Part model, mm, in its own coordinate system. A direction names the side the tool comes from. Give positions to 0.01 mm unless a question says otherwise; leave off trailing zeros. Write each loop counter-clockwise with the first axis right and the second up, starting at its lowest first coordinate (ties: lowest second). Pieces come first, ordered by that corner, then holes.
from build123d import *

# Parameters (mm, degrees)
SKETCH_1_R          = 4.75
EXTRUDE_1_DEPTH     = 7
SKETCH_2_R          = 6.5
EXTRUDE_2_DEPTH     = 1
SKETCH_3_R          = 6.5
EXTRUDE_3_DEPTH     = 1
SKETCH_4_R          = 1.5
CUT_EXTRUDE_1_DEPTH = 12
SKETCH_5_R          = 4
SKETCH_5_R_2        = 2
CUT_EXTRUDE_2_DEPTH = 0.5
SKETCH_6_R          = 4
SKETCH_6_R_2        = 2
CUT_EXTRUDE_3_DEPTH = 0.5


with BuildPart() as part:
    # 草图1 → 凸台-拉伸1 (new body)
    with BuildSketch(Plane.XY):
        Circle(SKETCH_1_R)
    extrude(amount=EXTRUDE_1_DEPTH)

    # 草图2 → 凸台-拉伸2 (add)
    with BuildSketch(Plane.XY.offset(7)):
        Circle(SKETCH_2_R)
    extrude(amount=EXTRUDE_2_DEPTH)

    # 草图3 → 凸台-拉伸3 (add)
    with BuildSketch(Plane(origin=(0, 0, 0), x_dir=(-1, 0, 0), z_dir=(0, 0, -1))):
        Circle(SKETCH_3_R)
    extrude(amount=EXTRUDE_3_DEPTH)

    # 草图4 → 切除-拉伸1 (cut)
    with BuildSketch(Plane(origin=(0, 0, -1), x_dir=(-1, 0, 0), z_dir=(0, 0, -1))):
        Circle(SKETCH_4_R)
    extrude(amount=-CUT_EXTRUDE_1_DEPTH, mode=Mode.SUBTRACT)

    # 草图5 → 切除-拉伸2 (cut)
    with BuildSketch(Plane(origin=(0, 0, -1), x_dir=(-1, 0, 0), z_dir=(0, 0, -1))):
        Circle(SKETCH_5_R)
        Circle(SKETCH_5_R_2, mode=Mode.SUBTRACT)
    extrude(amount=-CUT_EXTRUDE_2_DEPTH, mode=Mode.SUBTRACT)

    # 草图6 → 切除-拉伸3 (cut)
    with BuildSketch(Plane.XY.offset(8)):
        Circle(SKETCH_6_R)
        Circle(SKETCH_6_R_2, mode=Mode.SUBTRACT)
    extrude(amount=-CUT_EXTRUDE_3_DEPTH, mode=Mode.SUBTRACT)


solid = part.part
1) Drill centre lines: L1, parallel to Y at x = 0, z = -0.65; L2, parallel to Z at x = 3.75, y = -5; L3, parallel to Y at x = 0, z = 1. Where is each one in solid material? Low to high.
Check result:
L1: y = -6.5 to -4, -2 to -1.5, 1.5 to 2, 4 to 6.5
L2: z = -1 to 0, 7 to 8
L3: y = -4.75 to -1.5, 1.5 to 4.75
2) Saw through at C-C (x = 2.5). Write the cut outline in (y, z).
Check result:
outline: (-6, -1) - (-3.12, -1) - (-3.12, -0.5) - (3.12, -0.5) - (3.12, -1) - (6, -1) - (6, 0) - (4.04, 0) - (4.04, 7) - (6, 7) - (6, 8) - (3.12, 8) - (3.12, 7.5) - (-3.12, 7.5) - (-3.12, 8) - (-6, 8) - (-6, 7) - (-4.04, 7) - (-4.04, 0) - (-6, 0) - close
3) 3-axis set-ups, long thin cutter, end or side, ignore diameter. For faces 1 (the flat face through (0, -5, 0)), 2 (the flat face through (2, -1, -0.5)), 3 (the cylindrical face through (-0.434, -1.952, 7.754)): which of +Z, -Z, +X, -X, +Y, -Y reach the whole face in a straight line?
Check result:
face 1: none
face 2: -Z
face 3: +Z
4) Flat gauge pin, fed straight in: P1, Ø1.5, axis at y = 2, z = 3.5, coming from the -X side. Where does the tip first touch, or does it go through?
Check result:
P1: stops at x = -4.58
5) Mould opens along Z. For faces 4 (the flat face through (3, 3, 8)), 5 (the cylindrical face through (2.192, -4.214, 3.451)), 6 (the cylindrical face through (1.5, 0.07, 3.44)) say: +Z half, -Z half, draft (parallel to the pull), parting line (faces both ways), or undercut.
Check result:
face 4: +Z half
face 5: undercut
face 6: draft
6) Saw through at D-D (z = 5.5). Write the cut outline in (x, y).
Check result:
outline: circle Ø9.5 at (0, 0); hole circle Ø3 at (0, 0)
